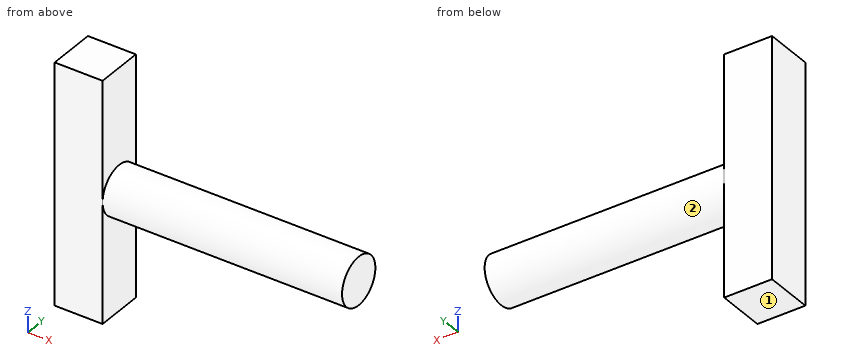
```python
from build123d import *

# Parameters (mm, degrees)
SKETCH1_W           = 25.4
SKETCH1_H           = 25.4
BOSS_EXTRUDE1_DEPTH = 127
SKETCH2_R           = 12.7
BOSS_EXTRUDE2_DEPTH = 127


with BuildPart() as part:
    # Sketch1 → Boss-Extrude1 (new body)
    with BuildSketch(Plane.XY):
        Rectangle(SKETCH1_W, SKETCH1_H)
    extrude(amount=BOSS_EXTRUDE1_DEPTH)

    # Sketch2 → Boss-Extrude2 (add)
    with BuildSketch(Plane(origin=(12.7, 0, 0), x_dir=(0, 0, -1), z_dir=(1, 0, 0))):
        with Locations(Location((-63.5, 0, 0), (0, 0, 270))):
            Circle(SKETCH2_R)
    extrude(amount=BOSS_EXTRUDE2_DEPTH)


solid = part.part
```
Build history of the part. All positions in model axes, mm. Face numbers are marked on the shaded views. A direction names the side the tool comes from. Round coordinates to 2 decimals unless told otherwise and drop trailing zeros. Loops run counter-clockwise (first coordinate to the right, second up) from the corner with the lowest first, then second, coordinate; pieces in that order, holes last.
Item 1: Saw through at C-C (z = 82). List the corners of the cut face in (x, y), then the cut area to 3 significant figures.
Item 2: Saw through at B-B (x = 94). List the corners of the cut face in (y, z).
Item 3: Which spindle directions (+Z, -Z, +X, -X, +Y, -Y) get a long thin tool onto all of the face, cutting with end or side? Do the marked faces 1 and 2. Say none if no direction does.
Item 4: Pin check, flat tips, straight feed: P1, Ø3, axis at y = 9.5, z = 98, coming from the +X side; P2, Ø6, axis at x = 102, z = 68.5, coming from the +Y side; P3, Ø1, axis at x = 55.5, y = 5.5, coming from the +Z side. Stop position of each tip, or through.
Item 5: Saw through at A-A (y = 0). List the corners of the cut face in (x, z), then the cut area to 3 significant figures.
Item 6: Drill centre lines: line 1 along Z through (x, y) = (38.5, 1); line 2 along X through (y, z) = (-7, 82.5); line 3 along Z through (x, y) = (63, 2). Where is each one in solid material? Low to high.
Worked answers:
1. outline: (-12.7, -12.7) - (12.7, -12.7) - (12.7, 12.7) - (-12.7, 12.7) - close
1. area: 645 mm2
2. outline: circle Ø25.4 at (0, 63.5)
3. face 1: -Z, +X, -X, +Y, -Y
3. face 2: +X
4. P1: stops at x = 12.7
4. P2: stops at y = 12.54
4. P3: stops at z = 75.17
5. outline: (-12.7, 0) - (12.7, 0) - (12.7, 50.8) - (139.7, 50.8) - (139.7, 76.2) - (12.7, 76.2) - (12.7, 127) - (-12.7, 127) - close
5. area: 6,450 mm2
6. line 1: z = 50.84 to 76.16
6. line 2: x = -12.7 to 12.7
6. line 3: z = 50.96 to 76.04
